Here's how the part is built. I have some questions about the finished solid (model axes, mm). Face numbers are marked on the shaded views. A direction names the side the tool comes from. Coordinates: 2 decimals unless noted, no trailing zeros. Write each loop counter-clockwise with the first axis right and the second up, starting at its lowest first coordinate (ties: lowest second). Pieces come first, ordered by that corner, then holes. Notation, with made-up numbers: (26.5, 49.5) - (83.5, 49.5) arc R31 cw to (83.5, 79.5) - close; hole circle Ø6 at (-21, 1). An arc over 180 degrees is marked (long way). Answer in a Markdown table with one row per item. Add a question column.
Item 1: I'm going to push flat-ended pins straight in: pin 1 (1.5 mm diameter, centred on x = -29, z = 4, fed in from +Y); pin 2 (5 mm diameter, centred on x = -18.5, y = 20.5, fed in from +Z); pin 3 (5.5 mm diameter, centred on y = 9, z = 6, fed in from +X). Where does each tip first touch, or does it pass through?
Item 2: We'd pull the mould along Y, two halves only. Please class the marked faces 5, 6 and 7: +Y half, -Y half, draft (parallel to the pull), parting line (faces both ways), or undercut.
Item 3: Imagine slicing it at A-A (x = -18). Please give me the cut outline in (y, z).
Item 4: Imagine slicing it at B-B (x = -28.5). Please give me the cut outline in (y, z), plus the area to 3 significant figures.
Item 5: Which directions (+Z, -Z, +X, -X, +Y, -Y) give clear straight access to the entire face, cutting with the end or side of a thin tool? Please do the marked faces 1, 2, 3 and 4.
Item 6: If I drill on probe 1 along Z at (x, y) = (-7, 27); probe 2 along Z at (x, y) = (-9.5, 31); probe 3 along Z at (x, y) = (-3.5, 37), over which ranges is the centre line in solid material (lowest first)? Write a range as from..to.
from build123d import *

# Parameters (mm, degrees)
SKETCH1_W                       = 30
SKETCH1_H                       = 30
BOSS_EXTRUDE1_DEPTH             = 50
CUT_EXTRUDE1_DEPTH              = 55.313902456
SKETCH3_W                       = 6
SKETCH3_H                       = 30
CUT_EXTRUDE2_DEPTH              = 55.313902456
SKETCH5_W                       = 30
SKETCH5_H                       = 30
BOSS_EXTRUDE2_DEPTH             = 25
F_45_DEGREE_EXTRUSION_CUT_DEPTH = 73.926037689
SKETCH11_R                      = 1.625
CUT_EXTRUDE7_DEPTH              = 10
CHAMFER1_SIZE                   = 2
FILLET1_R                       = 2
SKETCH16_R                      = 2.675
CUT_EXTRUDE10_DEPTH             = 10
CUT_EXTRUDE11_DEPTH             = 9.5
FILLET2_R                       = 0.5
FILLET3_R                       = 0.5
SKETCH19_W                      = 49
SKETCH19_H                      = 3
CUT_EXTRUDE12_DEPTH             = 71.710678119
SKETCH20_W                      = 6.753728314
SKETCH20_H                      = 6.253099935
CUT_EXTRUDE13_DEPTH             = 15
SKETCH22_R                      = 2.65
CUT_EXTRUDE14_DEPTH             = 51.035604398
SKETCH23_R                      = 5
CUT_EXTRUDE15_DEPTH             = 2.5
SKETCH24_W                      = 5
SKETCH24_H                      = 15
CUT_EXTRUDE16_DEPTH             = 4
SKETCH25_W                      = 5
SKETCH25_H                      = 12.094379765
BOSS_EXTRUDE3_DEPTH             = 2
CHAMFER2_SIZE                   = 2
SKETCH26_W                      = 2.5
SKETCH26_H                      = 5.5
CUT_EXTRUDE17_DEPTH             = 71.710678119
FILLET4_R                       = 0.5
CUT_EXTRUDE18_DEPTH             = 2


with BuildPart() as part:
    # Sketch1 → Boss-Extrude1 (new body)
    with BuildSketch(Plane(origin=(0, 0, 0), x_dir=(1, 0, 0), z_dir=(0, 1, 0))):
        Rectangle(SKETCH1_W, SKETCH1_H)
    extrude(amount=BOSS_EXTRUDE1_DEPTH)

    # Sketch2 → Cut-Extrude1 (cut, through all)
    with BuildSketch(Plane(origin=(0, 50, 0), x_dir=(1, 0, 0), z_dir=(0, 1, 0))):
        Polygon((-10.05, -2.5), (-10.05, -10.05), (10.05, -10.05), (10.05, 10.05), (-10.05, 10.05), (-10.05, 2.5), (-5.05, 2.5), (-5.05, -2.5), align=None)
    extrude(amount=-CUT_EXTRUDE1_DEPTH, mode=Mode.SUBTRACT)

    # Sketch3 → Cut-Extrude2 (cut, through all)
    with BuildSketch(Plane(origin=(0, 50, 0), x_dir=(1, 0, 0), z_dir=(0, 1, 0))):
        with Locations((12, 0)):
            Rectangle(SKETCH3_W, SKETCH3_H)
    extrude(amount=-CUT_EXTRUDE2_DEPTH, mode=Mode.SUBTRACT)

    # Sketch5 → Boss-Extrude2 (add)
    with BuildSketch(Plane.ZY.offset(15)):
        with Locations((0, 15)):
            Rectangle(SKETCH5_W, SKETCH5_H)
    extrude(amount=BOSS_EXTRUDE2_DEPTH)

    # Sketch7 → 45 degree extrusion cut (cut, through all)
    with BuildSketch(Plane(origin=(-40, 12.069825676, -23.451382923), x_dir=(-1, 0, 0), z_dir=(0, -0.42261826174069717, -0.9063077870366509))):
        Polygon((-25.1, -17.010685759), (-25.1, -24.560685759), (-17.55, -24.560685759), (-17.55, -19.560685759), (-12.55, -19.560685759), (-12.55, -24.560685759), (-5, -24.560685759), (-5, -17.010685759), (-10, -17.010685759), (-10, -14.510685759), (-20.1, -14.510685759), (-20.1, -17.010685759), align=None)
        Polygon((-25.1, -4.460685759), (-25.1, -12.010685759), (-20.1, -12.010685759), (-20.1, -14.510685759), (-10, -14.510685759), (-10, -12.010685759), (-5, -12.010685759), (-5, -4.460685759), (-12.55, -4.460685759), (-12.55, -9.460685759), (-17.55, -9.460685759), (-17.55, -4.460685759), align=None)
    extrude(amount=-F_45_DEGREE_EXTRUSION_CUT_DEPTH, mode=Mode.SUBTRACT)

    # Sketch11 → Cut-Extrude7 (cut)
    with BuildSketch(Plane(origin=(9, 0, 0), x_dir=(0, 0, -1), z_dir=(1, 0, 0))):
        with Locations((-12.525, 40)):
            Circle(SKETCH11_R)
        with Locations((12.525, 40)):
            Circle(SKETCH11_R)
        with Locations((12.525, 13)):
            Circle(SKETCH11_R)
        with Locations((-12.525, 13)):
            Circle(SKETCH11_R)
    extrude(amount=-CUT_EXTRUDE7_DEPTH, mode=Mode.SUBTRACT)

    # Chamfer1
    chamfer1_edges = [part.edges().sort_by_distance(p)[0] for p in [
        (-5.45, 0, -15),
        (-3, 50, -15),
        (-27.5, 30, -15),
        (-40, 15, -15),
        (-15, 40, -15),
        (-35, 0, -15),
    ]]
    chamfer(chamfer1_edges, length=CHAMFER1_SIZE)

    # Fillet1
    fillet1_edges = [part.edges().sort_by_distance(p)[0] for p in [
        (-15, 50, 1),
        (-15, 30, 1),
        (-40, 30, 1),
        (-40, 0, 1),
    ]]
    fillet(fillet1_edges, radius=FILLET1_R)

    # Sketch16 → Cut-Extrude10 (cut)
    with BuildSketch(Plane.ZY.offset(40)):
        with Locations((1, 7.415122828)):
            Circle(SKETCH16_R)
    extrude(amount=-CUT_EXTRUDE10_DEPTH, mode=Mode.SUBTRACT)

    # Sketch18 → Cut-Extrude11 (cut, symmetric)
    with BuildSketch(Plane.ZY.offset(25)):
        Polygon((9.950685103, 7.347750191), (5.606439218, 14.127716409), (-7.950685103, 7.482495466), (-3.606439218, 0.702529248), align=None)
    extrude(amount=CUT_EXTRUDE11_DEPTH, both=True, mode=Mode.SUBTRACT)

    # Fillet2
    fillet2_edges = [part.edges().sort_by_distance(p)[0] for p in [
        (-24.95, 0, -3.050682005),
    ]]
    fillet(fillet2_edges, radius=FILLET2_R)

    # Fillet3
    fillet3_edges = [part.edges().sort_by_distance(p)[0] for p in [
        (-24.95, 8.417171254, 15),
    ]]
    fillet(fillet3_edges, radius=FILLET3_R)

    # Sketch19 → Cut-Extrude12 (cut, through all)
    with BuildSketch(Plane.XY.offset(15)):
        with Locations((-15.5, 1.5)):
            Rectangle(SKETCH19_W, SKETCH19_H)
    extrude(amount=-CUT_EXTRUDE12_DEPTH, mode=Mode.SUBTRACT)


with BuildPart() as cut_extrude12_piece_1:
    # of the separate pieces the step leaves, piece 1, a body of its own (cut_extrude12_pieces)
    add(part.part.solids().sort_by_distance((-14.9, 3, 15))[0])

    # Sketch22 → Cut-Extrude14 (cut, through all)
    with BuildSketch(Plane(origin=(-25, 31.908299393, -7.624586929), x_dir=(1, 0, 0), z_dir=(3.142436568436473e-15, 0.8851034809979968, -0.46539427147874146))):
        with Locations(Location((0.022023463, 0.014340274, 0), (0, 0, 201.118214674))):
            Circle(SKETCH22_R)
    extrude(amount=-CUT_EXTRUDE14_DEPTH, mode=Mode.SUBTRACT)

    # Sketch23 → Cut-Extrude15 (cut)
    with BuildSketch(Plane(origin=(-25, 31.908299393, -7.624586929), x_dir=(1, 0, 0), z_dir=(3.142436568436473e-15, 0.8851034809979968, -0.46539427147874146))):
        with Locations((0.022023463, 0.014340274)):
            Circle(SKETCH23_R)
    extrude(amount=-CUT_EXTRUDE15_DEPTH, mode=Mode.SUBTRACT)

    # Sketch24 → Cut-Extrude16 (cut)
    with BuildSketch(Plane(origin=(0, 10.322187648, -4.813315149), x_dir=(1, 0, 0), z_dir=(0, -0.906307787036651, 0.4226182617406971))):
        with Locations((-24.95, 7.684747226)):
            Rectangle(SKETCH24_W, SKETCH24_H)
    extrude(amount=-CUT_EXTRUDE16_DEPTH, mode=Mode.SUBTRACT)

    # Sketch25 → Boss-Extrude3 (add)
    with BuildSketch(Plane.XZ.offset(-3)):
        with Locations((-37.5, 0.91772931)):
            Rectangle(SKETCH25_W, SKETCH25_H)
    extrude(amount=BOSS_EXTRUDE3_DEPTH)

    # Chamfer2
    chamfer2_edges = [cut_extrude12_piece_1.edges().sort_by_distance(p)[0] for p in [
        (-37.5, 1, -5.129460572),
        (-37.5, 1, 6.964919193),
    ]]
    chamfer(chamfer2_edges, length=CHAMFER2_SIZE - 0.0001)  # a hair under: the kernel refuses the full size

    # Sketch26 → Cut-Extrude17 (cut, through all)
    with BuildSketch(Plane.XY.offset(15)):
        with Locations((4, 40)):
            Rectangle(SKETCH26_W, SKETCH26_H)
        with Locations((4, 13)):
            Rectangle(SKETCH26_W, SKETCH26_H)
    extrude(amount=-CUT_EXTRUDE17_DEPTH, mode=Mode.SUBTRACT)

    # Fillet4
    fillet4_edges = [cut_extrude12_piece_1.edges().sort_by_distance(p)[0] for p in [
        (-32.5, 3, -14.481983196),
        (-24.95, 5.572058491, -15),
        (-17.4, 3, -14.481983196),
    ]]
    fillet(fillet4_edges, radius=FILLET4_R)

    # Mobious Logo → Cut-Extrude18 (cut)
    with BuildSketch(Plane(origin=(0, 0, 15), x_dir=(-1, 0, 0), z_dir=(0, 0, 1))):
        Polygon((-3.210868628, -32.348650408), (-3.210868628, -34.003716414), (7.056151005, -39.978785217), (7.056151005, -30.244752942), (5.33825141, -31.122174097), (5.33825141, -37.454108258), align=None)
        Polygon((1.978745121, -32.657222036), (0.744458608, -31.899818949), (9.188100437, -27.07488076), (9.188100437, -39.614109657), (7.533034431, -39.985072727), (7.533034431, -29.307901849), align=None)
        Polygon((4.840045674, -36.584497306), (-2.958400932, -31.899818949), (6.355467669, -26.569945368), (-2.958400932, -21.268123754), (4.840045674, -16.805452407), (4.840045674, -18.400245934), (-0.171524822, -21.268123754), (9.019468658, -26.5), (-0.416628352, -31.899818949), (4.840045674, -34.892125279), align=None)
        Polygon((-3.210868628, -20.791240329), (-3.210868628, -19.220330221), (7.056151005, -13.30136535), (7.056151005, -23.063449592), (5.33825141, -21.96942291), (5.33825141, -15.882146242), align=None)
        Polygon((0.744458608, -21.268123754), (9.188100437, -26.121113909), (9.188100437, -13.75019681), (7.533034431, -13.093877531), (7.533034431, -23.905008578), (1.915732347, -20.67645954), align=None)
    extrude(amount=-CUT_EXTRUDE18_DEPTH, mode=Mode.SUBTRACT)


with BuildPart() as cut_extrude12_piece_2:
    # of the separate pieces the step leaves, piece 2, a body of its own (cut_extrude12_pieces)
    add(part.part.solids().sort_by_distance((-27.45, 3, 15))[0])

    # Sketch20 → Cut-Extrude13 (cut)
    with BuildSketch(Plane.XY.offset(15)):
        with Locations((-25.201643275, 5.301831254)):
            Rectangle(SKETCH20_W, SKETCH20_H)
    extrude(amount=-CUT_EXTRUDE13_DEPTH, mode=Mode.SUBTRACT)


solid = cut_extrude12_piece_1.part
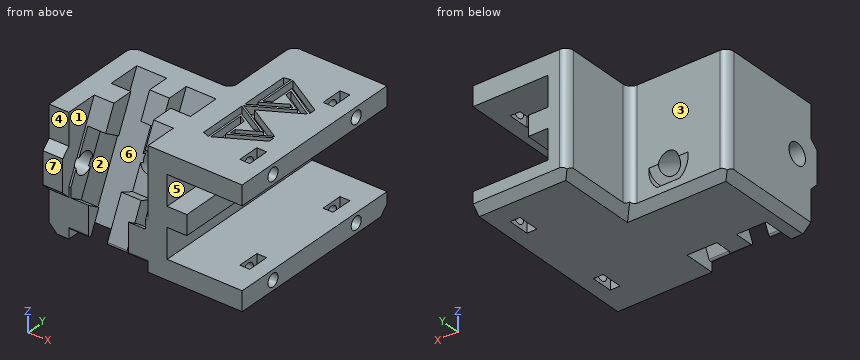
Here are the results:
| question | item | result |
|---|---|---|
| 1 | pin 1 | stops at y = 30 |
| 1 | pin 2 | stops at z = 10.54 |
| 1 | pin 3 | stops at x = -10.05 |
| 2 | face 5 | draft |
| 2 | face 6 | undercut |
| 2 | face 7 | -Y half |
| 3 | outline | (3, -12.23) arc R0.5 ccw to (3.95, -12.44) - (6.38, -7.24) - (3, -5.08) - close; (8.52, 9.2) - (12.77, 6.47) - (16.75, 15) - (11.23, 15) - close; (11.09, -15) - (28, -15) - (30, -13) - (30, 15) - (25.08, 15) - close |
| 4 | outline | (11.09, -15) - (28, -15) - (30, -13) - (30, -10.65) - (28.04, -9.62) - (30, -5.88) - (30, 15) - (25.08, 15) - close |
| 4 | area | 351 mm2 |
| 5 | face 1 | +Z, -Y |
| 5 | face 2 | none |
| 5 | face 3 | +Z, -Z, -X, +Y |
| 5 | face 4 | +Z, +X, -X, -Y |
| 6 | probe 1 | z = -15..-10.05, -2.5..2.5, 10.05..13 |
| 6 | probe 2 | z = -15..-10.05, -2.5..2.5, 10.05..15 |
| 6 | probe 3 | z = -15..-10.05, 10.05..13 |
